from build123d import *

# Parameters (mm, degrees)
F0_R     = 6.096
F1_DEPTH = 6.604
F2_R     = 3.175
F3_DEPTH = 19.05
F4_R     = 1.4103835631
F5_R     = 3.0660512242


with BuildPart() as f1:
    # F0 (on Top) → F1 (new body)
    with BuildSketch(Plane.XY):
        Circle(F0_R)
    extrude(amount=F1_DEPTH)

    # F2 (on face) → F3 (join)
    with BuildSketch(Plane.XY.offset(6.604)):
        Circle(F2_R)
    extrude(amount=F3_DEPTH)

    # F4
    f4_edges = [f1.edges().sort_by_distance(p)[0] for p in [
        (-6.096, 0, 6.604),
        (-3.175, 0, 6.604),
    ]]
    fillet(f4_edges, radius=F4_R)

    # F5
    f5_edges = [f1.edges().sort_by_distance(p)[0] for p in [
        (3.175, 0, 16.834192),
        (-3.175, 0, 8.014384),
        (-3.175, 0, 25.654),
    ]]
    fillet(f5_edges, radius=F5_R)


solid = f1.part
Can you work these out from the model? Positions are in its coordinate system, mm. A direction names the side the tool comes from. Give positions to 0.01 mm unless a question says otherwise; leave off trailing zeros. Order: outer loops, then holes, each group sorted by start corner. A loop starts at its lowest first (then second) coordinate and runs counter-clockwise, first axis right, second up. Notation, with made-up numbers: M 18,-38.75 L 32,-38.75 A21 ccw 32,-19.75 Z; hole C 48.25,-39.5 d7. An arc over 180 degrees is marked long. Use one line per item in the form item = value.
Item 1: Will these pins go through, and if not, where does the flat tip stop? pin 1 Ø6 at (x, z) = (-3.5, 13.5) entering from -Y; pin 2 Ø5 at (x, y) = (-3, 4.5) entering from +Z; pin 3 Ø1.5 at (x, y) = (2, -1) entering from +Z.
Values follow:
pin_1 = -3.14
pin_2 = 23.84
pin_3 = 25.33
Item 2: For faces 1 (the cylindrical face through (-0.69, -3.1, 15.2)), 2 (the cylindrical face through (-0.794, 6.044, 2.56)), which set-ups out of +Z, -Z, +X, -X, +Y, -Y let a thin tool reach every point of the face, with its end or its side?
Values follow:
face_1 = +Z
face_2 = +Z, -Z
Item 3: If we section it at B-B, the plane z = 4: Write out the boundary of the cut face in (x, y).
Values follow:
outline = C 0,0 d12.19
Item 4: If I drill on line 1 along Z through (x, y) = (2.75, 3.5); line 2 along X through (y, z) = (-1.75, 5.75); line 3 along Y through (x, z) = (1, 19.75), over which ranges is the centre line in solid material (lowest first)? Write a range as [from, to].
Values follow:
line_1 = [0, 6.61]
line_2 = [-5.72, 5.72]
line_3 = [-3.01, 3.01]
Item 5: If we section it at A-A, the plane z = 15.5: Write out the boundary of the cut face in (x, y) (3 decimals), and give its area (3 significant figures).
Values follow:
outline = C 0,0 d6.35
area = 31.7 mm^2
